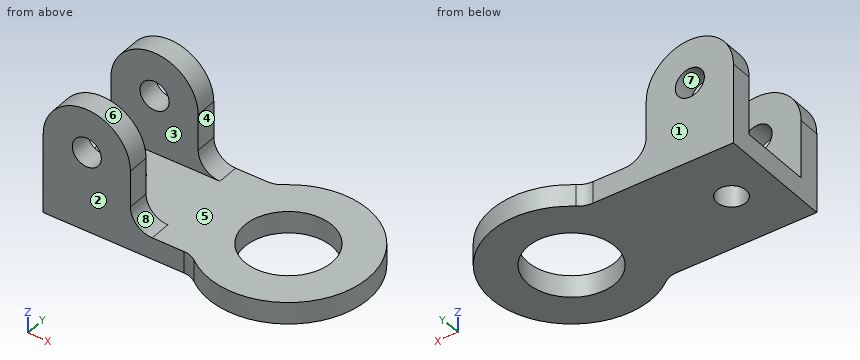
from build123d import *

# Parameters (mm, degrees)
F1_DEPTH  = 9.525
F2_R      = 19.05
F3_DEPTH  = 9.525
F4_W      = 38.1
F4_H      = 9.525
F5_DEPTH  = 25.4
F7_DEPTH  = 9.525
F8_R      = 6.35
F9_DEPTH  = 9.525
F10_R     = 19.05
F11_DEPTH = 9.525
F12_R     = 6.35
F13_DEPTH = 9.525
F14_R     = 6.35
F15_DEPTH = 25.4
F16_DEPTH = 9.525
F17_DEPTH = 9.525


with BuildPart() as f1:
    # F0 (on Top) → F1 (new body)
    with BuildSketch(Plane.XY):
        with BuildLine():
            Line((0, 50.8), (0, 0))
            Line((0, 0), (61.403693, 0))
            ThreePointArc((61.403693, 0), (64.521482, -0.524721), (67.295759, -2.041071))
            ThreePointArc((67.295759, -2.041071), (123.825, 25.4), (67.295759, 52.841071))
            ThreePointArc((67.295759, 52.841071), (64.521482, 51.324721), (61.403693, 50.8))
            Line((61.403693, 50.8), (0, 50.8))
        make_face()
    extrude(amount=F1_DEPTH)

    # F2 (on face) → F3 (cut)
    with BuildSketch(Plane.XY.offset(9.525)):
        with Locations((88.9, 25.4)):
            Circle(F2_R)
    extrude(amount=-F3_DEPTH, mode=Mode.SUBTRACT)

    # F4 (on face) → F5 (join)
    with BuildSketch(Plane.XY.offset(9.525)):
        with Locations((19.05, 4.7625)):
            Rectangle(F4_W, F4_H)
        with Locations((19.05, 46.0375)):
            Rectangle(F4_W, F4_H)
    extrude(amount=F5_DEPTH)

    # F6 (on face) → F7 (join)
    with BuildSketch(Plane(origin=(0, 50.8, 0), x_dir=(-1, 0, 0), z_dir=(0, 1, 0))):
        with BuildLine():
            ThreePointArc((-38.1, 34.925), (-19.05, 15.875), (0, 34.925))
            ThreePointArc((0, 34.925), (-19.05, 53.975), (-38.1, 34.925))
        make_face()
    extrude(amount=-F7_DEPTH)

    # F8 (on face) → F9 (cut)
    with BuildSketch(Plane(origin=(0, 50.8, 0), x_dir=(-1, 0, 0), z_dir=(0, 1, 0))):
        with Locations((-19.05, 34.925)):
            Circle(F8_R)
    extrude(amount=-F9_DEPTH, mode=Mode.SUBTRACT)

    # F10 (on face) → F11 (join)
    with BuildSketch(Plane.XZ):
        with Locations((19.05, 34.925)):
            Circle(F10_R)
    extrude(amount=-F11_DEPTH)

    # F12 (on face) → F13 (cut)
    with BuildSketch(Plane.XZ):
        with Locations((19.05, 34.925)):
            Circle(F12_R)
    extrude(amount=-F13_DEPTH, mode=Mode.SUBTRACT)

    # F14 (on face) → F15 (cut)
    with BuildSketch(Plane.XY.offset(9.525)):
        with Locations((19.05, 25.4)):
            Circle(F14_R)
    extrude(amount=-F15_DEPTH, mode=Mode.SUBTRACT)

    # F6 (on face) → F16 (join)
    with BuildSketch(Plane(origin=(0, 50.8, 0), x_dir=(-1, 0, 0), z_dir=(0, 1, 0))):
        with BuildLine():
            Line((-38.1, 9.525), (-38.1, 19.05))
            ThreePointArc((-38.1, 19.05), (-40.889808, 12.314808), (-47.625, 9.525))
            Line((-47.625, 9.525), (-38.1, 9.525))
        make_face()
    extrude(amount=-F16_DEPTH)

    # F10 (on face) → F17 (join)
    with BuildSketch(Plane.XZ):
        with BuildLine():
            ThreePointArc((47.625, 9.525), (40.889808, 12.314808), (38.1, 19.05))
            Line((38.1, 19.05), (38.1, 9.525))
            Line((38.1, 9.525), (47.625, 9.525))
        make_face()
    extrude(amount=-F17_DEPTH)


solid = f1.part
The listing builds one solid part. Answer for the finished solid, in the listing's coordinates (mm). Face numbers are marked on the shaded views. A direction names the side the tool comes from. Give positions to 0.01 mm unless a question says otherwise; leave off trailing zeros. Write each loop counter-clockwise with the first axis right and the second up, starting at its lowest first coordinate (ties: lowest second). Pieces come first, ordered by that corner, then holes.
1) Section B-B (x = 19.05) is taken. Write down the section's boundary in (y, z) (3 decimals), and give its area (3 significant figures).
2) Given P1, Ø1.5, axis at x = 49.5, y = 22, coming from the -Z side; P2, Ø22, axis at x = 18, z = 39, coming from the +Y side; P3, Ø2, axis at x = 23.5, z = 19.5, coming from the -Y side; P4, Ø11.5, axis at x = 19.05, z = 34.925, coming from the +Y side, each flat-ended and moving along its own axis, determine where each tip first touches the part or whether it passes through.
3) Find the intervals of material crossed by L1, parallel to Y at x = 19.05, z = 5; L2, parallel to Z at x = 19.05, y = 5.75 (3 decimals); L3, parallel to Z at x = 112.5, y = 22.5 (3 decimals), in increasing order.
4) Section C-C (x = 88.9) is taken. Write down the section's boundary in (y, z) (3 decimals), and give its area (3 significant figures).
5) Section A-A (y = 25.4) is taken. Write down the section's boundary in (x, z) (3 decimals).
6) For a pull along X with two mould halves and no side action, classify the marked faces 6, 7 and 8 as pulls with the +X half, pulls with the -X half, needs draft (parallel to the pull), parting line crosses it, or undercut.
7) Section D-D (z = 47) is taken. Write down the section's boundary in (x, y) (3 decimals), and give its area (3 significant figures).
8) A tool of negligible diameter and unlimited length cuts with its end or side. For the marked faces 1, 2, 3, 4 and 5, from which of +Z, -Z, +X, -X, +Y, -Y can it reach the whole face along a straight path? Write none if from no direction.
Response:
1. outline: (0, 0) - (19.05, 0) - (19.05, 9.525) - (9.525, 9.525) - (9.525, 28.575) - (0, 28.575) - close; (0, 41.275) - (9.525, 41.275) - (9.525, 53.975) - (0, 53.975) - close; (31.75, 0) - (50.8, 0) - (50.8, 28.575) - (41.275, 28.575) - (41.275, 9.525) - (31.75, 9.525) - close; (41.275, 41.275) - (50.8, 41.275) - (50.8, 53.975) - (41.275, 53.975) - close
1. area: 968 mm2
2. P1: stops at z = 0
2. P2: stops at y = 50.8
2. P3: stops at y = 0
2. P4: passes through
3. L1: y = 0 to 19.05, 31.75 to 50.8
3. L2: z = 0 to 28.575, 41.275 to 53.975
3. L3: z = 0 to 9.525
4. outline: (-9.525, 0) - (6.35, 0) - (6.35, 9.525) - (-9.525, 9.525) - close; (44.45, 0) - (60.325, 0) - (60.325, 9.525) - (44.45, 9.525) - close
4. area: 302 mm2
5. outline: (0, 0) - (12.7, 0) - (12.7, 9.525) - (0, 9.525) - close; (25.4, 0) - (69.85, 0) - (69.85, 9.525) - (25.4, 9.525) - close; (107.95, 0) - (123.825, 0) - (123.825, 9.525) - (107.95, 9.525) - close
6. face 6: parting line crosses it
6. face 7: undercut
6. face 8: pulls with the +X half
7. outline: (4.316, 0) - (33.784, 0) - (33.784, 9.525) - (4.316, 9.525) - close; (4.316, 41.275) - (33.784, 41.275) - (33.784, 50.8) - (4.316, 50.8) - close
7. area: 561 mm2
8. face 1: +Z, -Z, -X, +Y
8. face 2: +Z, -Z, -X, -Y
8. face 3: +Z, +X, -X
8. face 4: +Z, +X, +Y, -Y
8. face 5: +Z, +X
